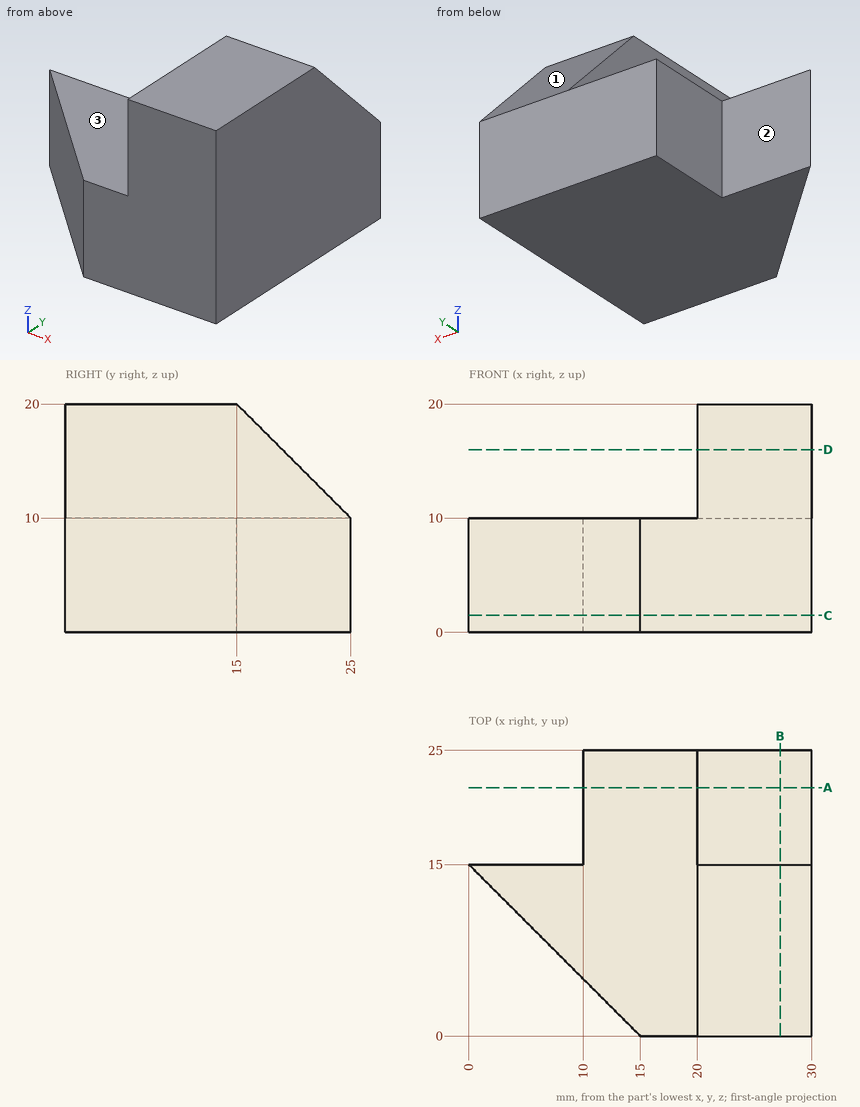
Check sheet for the drawn part. Datum: minimum x, y, z corner. Units: mm. A direction names the side the tool comes from. Round coordinates to 2 decimals unless told otherwise and drop trailing zeros. Order: outer loops, then holes, each group sorted by start corner. A loop starts at its lowest first (then second) coordinate and runs counter-clockwise, first axis right, second up.
(1) Scan lines: probe 1 along X at (y, z) = (22.75, 7.75); probe 2 along Z at (x, y) = (18, 20); probe 3 along X at (y, z) = (5.25, 17). Record each from-to range of solid material in increasing order.
(2) Cross-section at B-B, the plane x = 27.25. Enter the section's corners in (y, z), and give its area (3 significant figures).
(3) Cross-section at D-D, the plane z = 16. Enter the section's corners in (x, y).
(4) Access from +Z, -Z, +X, -X, +Y, -Y to the whole of each face (thin tool, end or side, straight path). Record for the marked faces 1, 2 and 3.
(5) Go/stop test with flat-tipped pins: P1, Ø3, axis at y = 4, z = 17.5, coming from the -X side; P2, Ø1, axis at x = 8, z = 6, coming from the -Y side; P3, Ø1.5, axis at y = 16, z = 3, coming from the -X side. Record where each tip stops, or that it passes through.
(6) Cross-section at C-C, the plane z = 1.5. Enter the section's corners in (x, y), and give its area (4 significant figures).
(7) Cross-section at A-A, the plane y = 21.75. Enter the section's corners in (x, z), and give its area (4 significant figures).
Check sheet entries:
1. probe 1: x = 10 to 30
1. probe 2: z = 0 to 10
1. probe 3: x = 20 to 30
2. outline: (0, 0) - (25, 0) - (25, 10) - (15, 20) - (0, 20) - close
2. area: 450 mm2
3. outline: (20, 0) - (30, 0) - (30, 19) - (20, 19) - close
4. face 1: +Z, +X, -X, +Y
4. face 2: +Z, -Z, -X, +Y
4. face 3: +Z, -X, +Y, -Y
5. P1: stops at x = 20
5. P2: stops at y = 6.5
5. P3: stops at x = 10
6. outline: (0, 15) - (15, 0) - (30, 0) - (30, 25) - (10, 25) - (10, 15) - close
6. area: 537.5 mm2
7. outline: (10, 0) - (30, 0) - (30, 13.25) - (20, 13.25) - (20, 10) - (10, 10) - close
7. area: 232.5 mm2
